For this review, use the dimensioned drawing (mm, ordinates from the lowest corner) and the shaded views. Round coordinates to 2 decimals unless told otherwise and drop trailing zeros. Loops run counter-clockwise (first coordinate to the right, second up) from the corner with the lowest first, then second, coordinate; pieces in that order, holes last. Notation, with made-up numbers: (-14.75, 10) -> (15.25, 10) arc R7 cw to (15.25, 21) -> close; hole circle Ø7 at (81.25, -24.5). An arc over 180 degrees is marked (long way). Write each question's results on one line, items separated by ' | '. Start each with the question number.
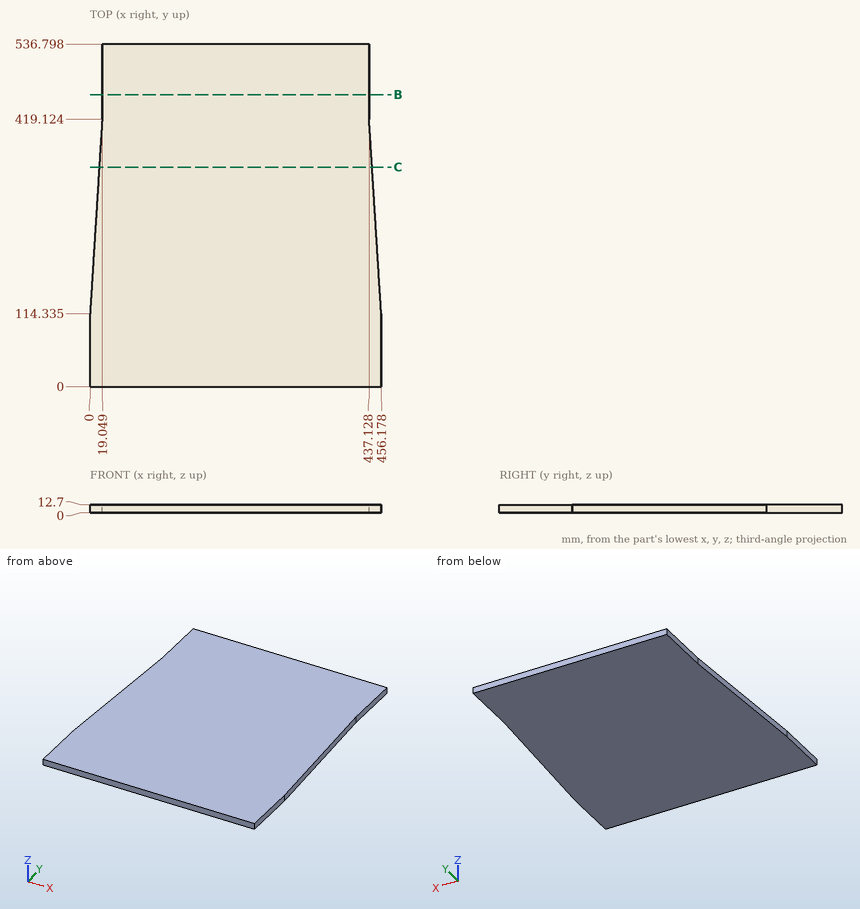
1) Take a section at C-C (y = 344). Write out the cut boundary in (x, z) (1 decimal).
2) To check wall thickness, follow line 1 (X direction, y = 475, z = 10.75); line 2 (X direction, y = 256.5, z = 11) (1 decimal). State the ranges of each line that lie inside material, in increasing order. Write a range as from..to.
3) Take a section at B-B (y = 457.5). Write out the cut boundary in (x, z).
4) Insertion check: pin 1 (4 mm diameter, centred on y = 453, z = 6.5, fed in from -X); pin 2 (5 mm diameter, centred on y = 247.5, z = 10.5, fed in from +X). Each pin has a flat end and moves straight along its axis. Give the tip position at first contact, or say it passes through.
Geometry check:
1) outline: (14.4, 0) -> (441.8, 0) -> (441.8, 12.7) -> (14.4, 12.7) -> close
2) line 1: x = 19.05..437.13 | line 2: x = 8.9..447.3
3) outline: (19.05, 0) -> (437.13, 0) -> (437.13, 12.7) -> (19.05, 12.7) -> close
4) pin 1: stops at x = 19.05 | pin 2: stops at x = 448.01
